from build123d import *

# Parameters (mm, degrees)
SKETCH_1_R          = 160
EXTRUDE_1_DEPTH     = 10
EXTRUDE_START       = 10
SKETCH_3_R          = 160
SKETCH_3_R_2        = 155
EXTRUDE_1_2_DEPTH   = 10
SKETCH_4_R          = 5
CUT_EXTRUDE_1_DEPTH = 228.156333832


with BuildPart() as part:
    # 草图1 → Extrude 1 (new body)
    with BuildSketch(Plane.XY):
        Circle(SKETCH_1_R)
    extrude(amount=EXTRUDE_1_DEPTH)

    # 草图3 → Extrude 1 2 (add)
    with BuildSketch(Plane(origin=(0, 0, 0), x_dir=(-1, 0, 0), z_dir=(0, 0, -1)).offset(EXTRUDE_START)):
        Circle(SKETCH_3_R)
        Circle(SKETCH_3_R_2, mode=Mode.SUBTRACT)
    extrude(amount=-EXTRUDE_1_2_DEPTH)

    # 草图4 → 切除-拉伸1 (cut, through all)
    with BuildSketch(Plane.XY.offset(10)):
        Circle(SKETCH_4_R)
    extrude(amount=-CUT_EXTRUDE_1_DEPTH, mode=Mode.SUBTRACT)


solid = part.part
Could you check a few things on this model? Use its own coordinates, in mm. A direction names the side the tool comes from. Round coordinates to 2 decimals unless told otherwise and drop trailing zeros. Write each loop counter-clockwise with the first axis right and the second up, starting at its lowest first coordinate (ties: lowest second). Pieces come first, ordered by that corner, then holes. Notation, with made-up numbers: (39, -25) - (74, -25) arc R9 cw to (74, -10) - close; hole circle Ø1 at (-27, -10). An arc over 180 degrees is marked (long way). Use a Markdown table: item, result.
Q1. I want a section at D-D (x = -57). List the corners of the cut face in (y, z) for me.
Output values:
| item | result |
|---|---|
| outline | (-149.5, -10) - (-144.14, -10) - (-144.14, 0) - (144.14, 0) - (144.14, -10) - (149.5, -10) - (149.5, 10) - (-149.5, 10) - close |
Q2. For pin 1 (10 mm diameter, centred on x = 83.5, z = -5, fed in from -Y); pin 2 (2 mm diameter, centred on y = 111, z = -4, fed in from -X); pin 3 (1 mm diameter, centred on x = -113, y = -1, fed in from -Z), each with a flat end and sliding along its axis, tell me the tip position at first contact or that it passes through.
Output values:
| item | result |
|---|---|
| pin 1 | y = -139.42 |
| pin 2 | x = -116.19 |
| pin 3 | z = 0 |
Q3. I want a section at C-C (z = -3). List the corners of the cut face in (x, y) for me, plus the area to 3 significant figures.
Output values:
| item | result |
|---|---|
| outline | circle Ø320 at (0, 0); hole circle Ø310 at (0, 0) |
| area | 4,950 mm2 |
Q4. For faces 1 (the cylindrical face through (-1.08, -4.88, 5.07)), 2 (the flat face through (-2, -32, 0)), which set-ups out of +Z, -Z, +X, -X, +Y, -Y let a thin tool reach every point of the face, with its end or its side?
Output values:
| item | result |
|---|---|
| face 1 | +Z, -Z |
| face 2 | -Z |
Q5. I want a section at A-A (x = 0). List the corners of the cut face in (y, z) for me.
Output values:
| item | result |
|---|---|
| outline | (-160, -10) - (-155, -10) - (-155, 0) - (-5, 0) - (-5, 10) - (-160, 10) - close; (5, 0) - (155, 0) - (155, -10) - (160, -10) - (160, 10) - (5, 10) - close |
Q6. Thinking about a two-plate mould opening in Y: for faces 3 (the cylindrical face through (33.601, -151.314, -5.07)), 4 (the flat face through (84, 131, -10)), which applies, released by +Y, released by -Y, zero draft, split by the parting line, or undercut?
Output values:
| item | result |
|---|---|
| face 3 | undercut |
| face 4 | zero draft |
Q7. Please list where these lines run through material, in increasing order: L1, parallel to Y at x = 0, z = -4; L2, parallel to Y at x = 0, z = 2.5; L3, parallel to Z at x = -20.5, y = -29.5.
Output values:
| item | result |
|---|---|
| L1 | -160 to -155, 155 to 160 |
| L2 | -160 to -5, 5 to 160 |
| L3 | 0 to 10 |
